Autodesk Inventor part; units mm, degrees
ref_plane "YZ Plane" through (0, 0, 0) normal (1, 0, 0) x (0, 1, 0)
ref_plane "XZ Plane" through (0, 0, 0) normal (0, 1, 0) x (-1, 0, 0)
ref_plane "XY Plane" through (0, 0, 0) normal (0, 0, 1) x (1, 0, 0)
sketch "Boceto1" plane through (0, 0, 0) normal (0, 1, 0) x (-1, 0, 0)
  circle A0 centre (0, 0) radius 12.7
  circle A1 centre (0, 0) radius 15.875
  dimension "d0" = 25.4
  dimension "d1" = 31.75
extrude "Extrusión1" add sketch "Boceto1" along normal blind 4.7
sketch "Boceto2" plane through (0, 4.7, 0) normal (0, 1, 0) x (1, 0, 0)
  circle A0 centre (0, 0) radius 12.7
  dimension "d4" = 25.4
extrude "Extrusión2" add sketch "Boceto2" against normal blind 38.8
hole "Agujero1" at (0.5939, -34.1, -0.5568) direction (0, 1, 0) diameter 4 depth 8 counterbore diameter 10.2 counterbore depth 0.5
thread "Rosca1"
properties part number "post"
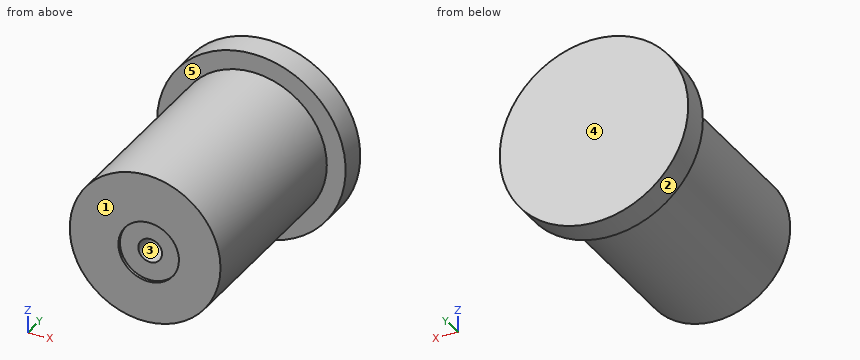
Check sheet for the modelled part. Datum: model origin and axes. Units: mm. Face numbers are marked on the shaded views. A direction names the side the tool comes from. Coordinates: 2 decimals unless noted, no trailing zeros. Order: outer loops, then holes, each group sorted by start corner. A loop starts at its lowest first (then second) coordinate and runs counter-clockwise, first axis right, second up. Notation, with made-up numbers: M -8,39.25 L 13,39.25 A20 cw 13,57.25 Z; hole C -29,-24 d6. An arc over 180 degrees is marked long. One line per question, with ' | ' between items. Start each with the question number.
Item 1: Sectioned sample at B-B on z = 0. Record the cut outline in (x, y) (3 decimals).
Item 2: Sectioned sample at D-D on x = -10. Record the cut outline in (y, z), and give its area (3 significant figures).
Item 3: Access from +Z, -Z, +X, -X, +Y, -Y to the whole of each face (thin tool, end or side, straight path). Record for the marked faces 4 and 5.
Item 4: Sectioned sample at A-A on x = 0. Record the cut outline in (y, z) (1 decimal), and give its area (3 significant figures).
Item 5: Gauge pin test, flat ends, axial feed: P1, Ø6, axis at x = 0.59, z = -0.56, coming from the -Y side; P2, Ø1.5, axis at y = -1.5, z = 5, coming from the +X side; P3, Ø1, axis at x = -12.5, z = 6, coming from the -Y side. Record the tip position at first contact, or that the pin passes through.
Item 6: Material ranges on line 1 (Y direction, x = -14, z = -3); line 2 (Z direction, x = -0.5, y = -26); line 3 (Z direction, x = -11, y = -12), recorded low to high.
Item 7: Sectioned sample at C-C on y = -5.5. Record the cut outline in (x, z).
Item 8: Mould release check, pull along X, two halves, no side actions. Record for the marked faces 1, 2 and 3: pulls with the +X half, pulls with the -X half, needs draft (parallel to the pull), parting line crosses it, or undercut.
Answer below:
1) outline: M -15.875,0 L -12.7,0 L -12.7,-34.1 L -4.476,-34.1 L -4.476,-33.6 L -1.327,-33.6 L -1.327,-26.1 L 2.515,-26.1 L 2.515,-33.6 L 5.663,-33.6 L 5.663,-34.1 L 12.7,-34.1 L 12.7,0 L 15.875,0 L 15.875,4.7 L -15.875,4.7 Z
2) outline: M -34.1,-7.83 L 0,-7.83 L 0,-12.33 L 4.7,-12.33 L 4.7,12.33 L 0,12.33 L 0,7.83 L -34.1,7.83 Z | area: 650 mm^2
3) face 4: +Z, -Z, +X, -X, +Y | face 5: -Y
4) outline: M -34.1,-12.7 L 0,-12.7 L 0,-15.9 L 4.7,-15.9 L 4.7,15.9 L 0,15.9 L 0,12.7 L -34.1,12.7 L -34.1,4.5 L -33.6,4.5 L -33.6,1.4 L -26.1,1.4 L -26.1,-2.5 L -33.6,-2.5 L -33.6,-5.6 L -34.1,-5.6 Z | area: 982 mm^2
5) P1: stops at y = -33.6 | P2: stops at x = 11.97 | P3: stops at y = 0
6) line 1: y = 0 to 4.7 | line 2: z = -12.69 to 12.69 | line 3: z = -6.35 to 6.35
7) outline: C 0,0 d25.4
8) face 1: needs draft | face 2: parting line crosses it | face 3: undercut
